Could you check a few things on this model? Use its own coordinates, in mm. Round coordinates to 2 decimals unless told otherwise and drop trailing zeros. Loops run counter-clockwise (first coordinate to the right, second up) from the corner with the lowest first, then second, coordinate; pieces in that order, holes last. Notation, with made-up numbers: (30.25, -36.5) -> (54.25, -36.5) arc R26 cw to (54.25, -10.5) -> close; hole circle Ø11 at (-32.75, 53). An arc over 180 degrees is marked (long way). One line per item, written item: value.
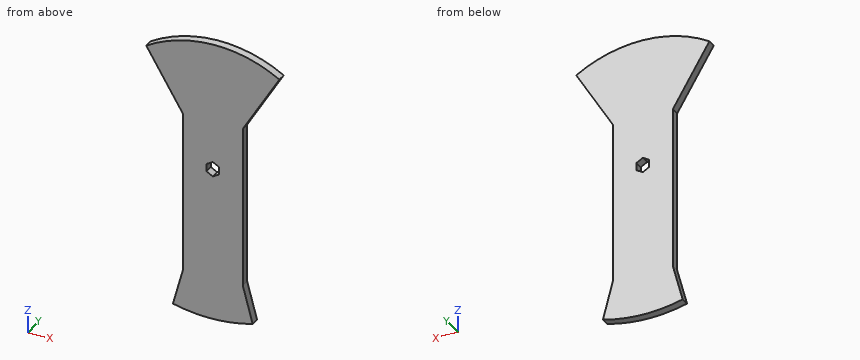
```python
from build123d import *

# Parameters (mm, degrees)
BOSS_EXTRUDE1_DEPTH = 3.175
CUT_EXTRUDE1_REACH  = 126.672


with BuildPart() as part:
    # Sketch1 → Boss-Extrude1 (new, symmetric)
    with BuildSketch(Plane(origin=(0, 0, 0), x_dir=(1, 0, 0), z_dir=(0, 1, 0))):
        with BuildLine():
            Line((-22.225, 82.944829198), (-22.225, -36.659057496))
            Line((-22.225, -36.659057496), (-49.38024545, -81.450315281))
            ThreePointArc((-49.38024545, -81.450315281), (0, -95.25), (49.38024545, -81.450315281))
            Line((49.38024545, -81.450315281), (22.225, -36.659057496))
            Line((22.225, -36.659057496), (22.225, 82.944829198))
            Line((22.225, 82.944829198), (29.583016855, 110.405321945))
            ThreePointArc((29.583016855, 110.405321945), (0, 114.3), (-29.583016855, 110.405321945))
            Line((-29.583016855, 110.405321945), (-22.225, 82.944829198))
        make_face()
    extrude(amount=BOSS_EXTRUDE1_DEPTH, both=True)

    # Sketch2 → Cut-Extrude1 (cut, up to next)
    with BuildSketch(Plane(origin=(0, 3.175, 0), x_dir=(1, 0, 0), z_dir=(0, 1, 0)), mode=Mode.PRIVATE) as cut_extrude1_sk1:
        Polygon((4.7625, -2.749630657), (4.7625, 2.749630657), (0, 5.499261314), (-4.7625, 2.749630657), (-4.7625, -2.749630657), (0, -5.499261314), align=None)
    cut_extrude1_tool1 = extrude(cut_extrude1_sk1.sketch, amount=-CUT_EXTRUDE1_REACH, mode=Mode.PRIVATE) & part.part
    add(cut_extrude1_tool1.solids().sort_by_distance((0, 3.175, 0))[0], mode=Mode.SUBTRACT)


solid = part.part
```
(1) Imagine slicing it at C-C on x = 37. Write out the boundary of the cut face in (y, z) (3 decimals).
Results below:
outline: (-3.175, 61.03) -> (3.175, 61.03) -> (3.175, 87.77) -> (-3.175, 87.77) -> close
(2) Imagine slicing it at B-B on z = -44. Write out the boundary of the cut face in (x, y) (3 decimals), then the cut area to 3 significant figures.
Results below:
outline: (-22.225, -3.175) -> (22.225, -3.175) -> (22.225, 3.175) -> (-22.225, 3.175) -> close
area: 282 mm²
(3) For pin 1 Ø1.6 at (y, z) = (1, -0.5) entering from +X (3 decimals); pin 2 Ø1.5 at (x, z) = (-22.5, -32.5) entering from -Y (3 decimals); pin 3 Ø1.5 at (x, y) = (-35, -0.5) entering from -Z; pin 4 Ø1.6 at (y, z) = (-1, 0) entering from -X (3 decimals), each with a flat end and sliding along its axis, tell me the tip position at first contact or that it passes through.
Results below:
pin 1: stops at x = 22.225
pin 2: stops at y = -3.175
pin 3: stops at z = 56.49
pin 4: stops at x = -22.225
(4) Please list where these lines run through material, in increasing order: L1, parallel to X at y = 3, z = -7.5 (3 decimals); L2, parallel to Z at x = -2, y = -2; L3, parallel to Z at x = -5.5, y = -1.
Results below:
L1: x = -22.225 to 22.225
L2: z = -114.28 to -4.34, 4.34 to 95.23
L3: z = -114.17 to 95.09
